```python
from build123d import *

# Parameters (mm, degrees)
BOSS_EXTRUDE1_DEPTH      = 88.9
CUT_EXTRUDE2_DEPTH       = 241.232341963
CUT_EXTRUDE2_DEPTH_BACK  = 241.232341963
SKETCH3_R                = 28.575
CUT_EXTRUDE5_DEPTH       = 28.575
CUT_EXTRUDE6_DEPTH       = 243.134084755
CUT_EXTRUDE6_DEPTH_BACK  = 243.134084755
SKETCH4_R                = 12.7
CUT_EXTRUDE7_DEPTH       = 261.369359036
CUT_EXTRUDE7_DEPTH_BACK  = 261.369359036
CUT_EXTRUDE8_DEPTH       = 261.369359036
CUT_EXTRUDE8_DEPTH_BACK  = 12.7
SKETCH6_R                = 9.525
SKETCH7_R                = 6.35
CUT_EXTRUDE9_DEPTH       = 12.7
SKETCH12_R               = 13.5
CUT_EXTRUDE13_DEPTH      = 3.175
CUT_EXTRUDE14_DEPTH      = 253.187753717
CUT_EXTRUDE14_DEPTH_BACK = 253.187753717
SKETCH14_R               = 1.5875
CUT_EXTRUDE15_DEPTH      = 261.369359036
CUT_EXTRUDE15_DEPTH_BACK = 261.369359036
SKETCH15_W               = 158.75
SKETCH15_H               = 174.625
SKETCH16_R               = 6.35
BOSS_EXTRUDE2_DEPTH      = 12.7
CHAMFER1_SIZE            = 1.5875


with BuildPart() as part:
    # Sketch1 → Boss-Extrude1 (new body)
    with BuildSketch(Plane.XY):
        Polygon((0, 0), (0, -174.625), (171.45, -174.625), (171.45, 0), (158.75, 0), (158.75, -142.875), (12.7, -142.875), (12.7, 0), align=None)
    extrude(amount=BOSS_EXTRUDE1_DEPTH)

    # Sketch2 → Cut-Extrude2 (cut, two sides: drawn at the far end of the back side and taken through both)
    with BuildSketch(Plane(origin=(0, -142.875, 0), x_dir=(1, 0, 0), z_dir=(0, 1, 0)).offset(-CUT_EXTRUDE2_DEPTH_BACK)):
        Polygon((158.75, 0), (12.7, 0), (12.7, -25.4), (85.724999876, -25.4), (158.75, -25.4), align=None)
    extrude(amount=CUT_EXTRUDE2_DEPTH + CUT_EXTRUDE2_DEPTH_BACK, mode=Mode.SUBTRACT)

    # Sketch3 → Cut-Extrude5 (cut)
    with BuildSketch(Plane.XZ.offset(174.625)):
        with Locations((85.725, 57.15)):
            Circle(SKETCH3_R)
    extrude(amount=-CUT_EXTRUDE5_DEPTH, mode=Mode.SUBTRACT)

    # Sketch4 → Cut-Extrude6 (cut, two sides: drawn at the far end of the back side and taken through both)
    with BuildSketch(Plane.XZ.offset(146.05).offset(-CUT_EXTRUDE6_DEPTH_BACK)):
        with Locations((85.725, 57.15)):
            Circle(SKETCH4_R)
    extrude(amount=CUT_EXTRUDE6_DEPTH + CUT_EXTRUDE6_DEPTH_BACK, mode=Mode.SUBTRACT)

    # Sketch5 → Cut-Extrude7 (cut, two sides: drawn at the far end of the back side and taken through both)
    with BuildSketch(Plane(origin=(171.45, 0, 0), x_dir=(0, 0, -1), z_dir=(1, 0, 0)).offset(-CUT_EXTRUDE7_DEPTH_BACK)):
        with BuildLine():
            Line((0, -174.625), (0, -114.3))
            ThreePointArc((0, -114.3), (-0.597344099, -119.776153781), (-2.361280333, -124.994736842))
            Line((-2.361280333, -124.994736842), (-25.4, -174.625))
            Line((-25.4, -174.625), (0, -174.625))
        make_face()
        with BuildLine():
            Line((-39.269490456, -98.025866748), (-71.745289975, -22.119448379))
            ThreePointArc((-71.745289975, -22.119448379), (-70.400400796, -7.131859618), (-57.149999966, 0))
            Line((-57.149999966, 0), (-88.9, 0))
            Line((-88.9, 0), (-88.9, -142.875))
            Line((-88.9, -142.875), (-50.8, -142.875))
            Line((-50.8, -142.875), (-39.583234749, -118.711720996))
            ThreePointArc((-39.583234749, -118.711720996), (-37.224875429, -108.402184034), (-39.269490456, -98.025866748))
        make_face()
        with BuildLine():
            Line((0, 0), (-57.149999966, 0))
            ThreePointArc((-57.149999966, 0), (-48.406859618, -2.624599204), (-42.554710025, -9.630551621))
            Line((-42.554710025, -9.630551621), (-2.047536041, -104.308882594))
            ThreePointArc((-2.047536041, -104.308882594), (-0.51714863, -109.200616928), (0, -114.3))
            Line((0, -114.3), (0, 0))
        make_face()
    extrude(amount=CUT_EXTRUDE7_DEPTH + CUT_EXTRUDE7_DEPTH_BACK, mode=Mode.SUBTRACT)

    # Sketch6 → Cut-Extrude8 (cut, two sides: drawn at the far end of the back side and taken through both)
    with BuildSketch(Plane(origin=(171.45, 0, 0), x_dir=(0, 0, -1), z_dir=(1, 0, 0)).offset(-CUT_EXTRUDE8_DEPTH_BACK)):
        with Locations(Location((-57.15, -15.875, 0), (0, 0, 90))):
            Circle(SKETCH6_R)
    extrude(amount=CUT_EXTRUDE8_DEPTH + CUT_EXTRUDE8_DEPTH_BACK, mode=Mode.SUBTRACT)

    # Sketch7 → Cut-Extrude9 (cut)
    with BuildSketch(Plane(origin=(12.7, 0, 0), x_dir=(0, 0, -1), z_dir=(1, 0, 0))):
        with Locations((-57.15, -15.875)):
            Circle(SKETCH7_R)
    extrude(amount=-CUT_EXTRUDE9_DEPTH, mode=Mode.SUBTRACT)

    # Sketch12 → Cut-Extrude13 (cut)
    with BuildSketch(Plane(origin=(12.7, 0, 0), x_dir=(0, 0, -1), z_dir=(1, 0, 0))):
        with Locations((-57.15, -15.875)):
            Circle(SKETCH12_R)
    extrude(amount=-CUT_EXTRUDE13_DEPTH, mode=Mode.SUBTRACT)

    # Sketch14 → Cut-Extrude14 (cut, two sides: drawn at the far end of the back side and taken through both)
    with BuildSketch(Plane(origin=(12.7, 0, 0), x_dir=(0, 0, -1), z_dir=(1, 0, 0)).offset(-CUT_EXTRUDE14_DEPTH_BACK)):
        with Locations((-53.770765225, -24.780413934)):
            Circle(SKETCH14_R)
        with Locations((-66.551932086, -14.348796194)):
            Circle(SKETCH14_R)
        with Locations((-51.12730269, -8.495789872)):
            Circle(SKETCH14_R)
    extrude(amount=CUT_EXTRUDE14_DEPTH + CUT_EXTRUDE14_DEPTH_BACK, mode=Mode.SUBTRACT)

    # Sketch15 → Cut-Extrude15 (cut, two sides: drawn at the far end of the back side and taken through both)
    with BuildSketch(Plane.XY.offset(88.9).offset(-CUT_EXTRUDE15_DEPTH_BACK)):
        with Locations((92.075, -87.3125)):
            Rectangle(SKETCH15_W, SKETCH15_H)
    extrude(amount=CUT_EXTRUDE15_DEPTH + CUT_EXTRUDE15_DEPTH_BACK, mode=Mode.SUBTRACT)

    # Sketch16 → Boss-Extrude2 (add)
    with BuildSketch(Plane(origin=(12.7, 0, 0), x_dir=(0, 0, -1), z_dir=(1, 0, 0))):
        with Locations(Location((-76.2, -158.75, 0), (0, 0, 180))):
            Circle(SKETCH16_R)
        with Locations(Location((-38.1, -158.75, 0), (0, 0, 180))):
            Circle(SKETCH16_R)
    extrude(amount=BOSS_EXTRUDE2_DEPTH)

    # Chamfer1
    chamfer1_edges = [part.edges().sort_by_distance(p)[0] for p in [
        (25.4, -158.75, 69.85),
        (25.4, -158.75, 31.75),
    ]]
    chamfer(chamfer1_edges, length=CHAMFER1_SIZE)


solid = part.part
```
Check sheet for the modelled part. Datum: model origin and axes. Units: mm. A direction names the side the tool comes from. Coordinates: 2 decimals unless noted, no trailing zeros. Loops run counter-clockwise (first coordinate to the right, second up) from the corner with the lowest first, then second, coordinate; pieces in that order, holes last.
1) Sectioned sample at C-C (z = 61.5). Record the boundary of the cut face in (x, y) (3 decimals), and give its area (3 significant figures).
2) Gauge pin test, flat ends, axial feed: pin 1 (10 mm diameter, centred on y = -18, z = 56, fed in from +X) (3 decimals); pin 2 (4 mm diameter, centred on x = 7, z = 59.5, fed in from +Y); pin 3 (21.5 mm diameter, centred on y = -10.5, z = 53.5, fed in from +X); pin 4 (2.5 mm diameter, centred on y = -24.78, z = 53.77, fed in from -X) (3 decimals). Record the tip position at first contact, or that the pin passes through.
3) Material ranges on probe 1 along Y at (x, z) = (7, 57.15) (3 decimals); probe 2 along X at (y, z) = (-23, 59) (3 decimals); probe 3 along Y at (x, z) = (10.3, 57.15) (3 decimals), recorded low to high.
4) Access from +Z, -Z, +X, -X, +Y, -Y to the whole of each face (thin tool, end or side, straight path). Record for faces 1 (the face through (25.4, -159, 76)), 2 (the face through (11.135, -11.82, 44.273)), 3 (the face through (6.26, -130.96, 45.27)).
5) Sectioned sample at A-A (z = 76.2). Record the boundary of the cut face in (x, y) (1 decimal), and give its area (3 significant figures).
6) Sectioned sample at D-D (y = -158.75). Record the boundary of the cut face in (x, z), and give its area (3 significant figures).
7) Sectioned sample at B-B (x = 2). Count the separate pieces of the cut face and the enclosed holes in it, and give its area (3 significant figures).
8) Release check for a two-part mould opening along Z. For faces 4 (the face through (4.83, -19.74, 62.19)), 5 (the face through (6, -174.625, 57)), 6 (the face through (6.26, -60.6, 55.28)) record: released by +Z, released by -Z, zero draft, split by the parting line, or undercut.
Check sheet entries:
1. outline: (0, -174.625) - (12.7, -174.625) - (12.7, -142.875) - (0, -142.875) - close; (0, -46.066) - (12.7, -46.066) - (12.7, -28.655) - (9.525, -28.655) - (9.525, -20.501) - (0, -20.501) - close; (0, -11.249) - (9.525, -11.249) - (9.525, -3.095) - (12.7, -3.095) - (12.7, -0.608) - (0, -0.608) - close
1. area: 811 mm2
2. pin 1: stops at x = 9.525
2. pin 2: stops at y = 0
2. pin 3: stops at x = 12.7
2. pin 4: passes through
3. probe 1: y = -174.625 to -142.875, -56.233 to -22.225, -9.525 to 0
3. probe 2: x = 0 to 9.525
3. probe 3: y = -174.625 to -142.875, -56.233 to -29.375, -2.375 to 0
4. face 1: +Z, -Z, +X, +Y, -Y
4. face 2: +X
4. face 3: +Z, +X, -X
5. outline: (0, -174.6) - (12.7, -174.6) - (12.7, -165.1) - (23.8, -165.1) - (25.4, -163.5) - (25.4, -154) - (23.8, -152.4) - (12.7, -152.4) - (12.7, -142.9) - (0, -142.9) - close
5. area: 562 mm2
6. outline: (0, 18.03) - (12.7, 18.03) - (12.7, 31.75) - (23.81, 31.75) - (25.4, 33.34) - (25.4, 42.86) - (23.81, 44.45) - (12.7, 44.45) - (12.7, 69.85) - (23.81, 69.85) - (25.4, 71.44) - (25.4, 80.96) - (23.81, 82.55) - (12.7, 82.55) - (12.7, 88.9) - (0, 88.9) - close
6. area: 1,220 mm2
7. separate pieces: 1
7. enclosed holes: 4
7. area: 7,060 mm2
8. face 4: undercut
8. face 5: zero draft
8. face 6: released by +Z
